Geometry: see drawing. Coordinates: mm, zero at the bounding-box minimum. A direction names the side the tool comes from. Coordinates: 2 decimals unless noted, no trailing zeros. Loops run counter-clockwise (first coordinate to the right, second up) from the corner with the lowest first, then second, coordinate; pieces in that order, holes last.
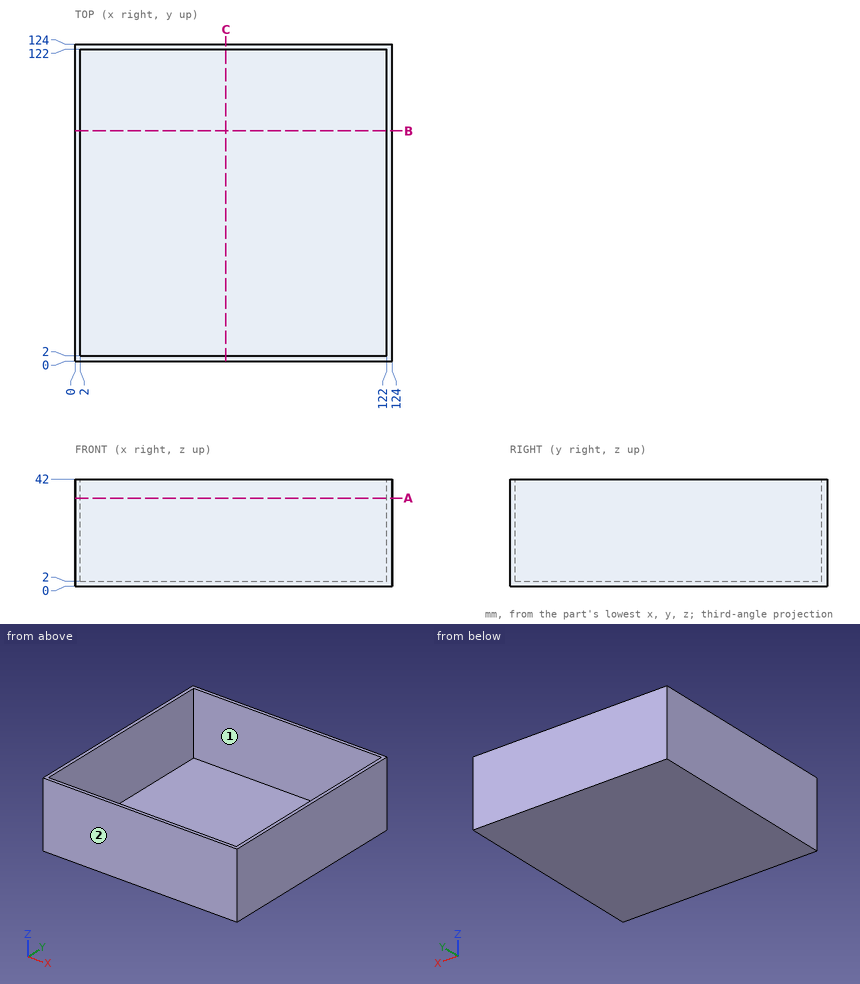
Item 1: Reachability of the marked faces 1 and 2 from +Z, -Z, +X, -X, +Y, -Y: full face, straight path, thin tool, end or side. Return the list, or none.
Result:
face 1: +Z
face 2: +Z, -Z, +X, -X, -Y
Item 2: Section query A-A (z = 34.5). Output: boundary loops of the cut face in (x, y), then the cut area to 3 significant figures.
Result:
outline: (0, 0) - (124, 0) - (124, 124) - (0, 124) - close; hole (2, 2) - (122, 2) - (122, 122) - (2, 122) - close
area: 976 mm2
Item 3: Section query B-B (y = 90). Output: boundary loops of the cut face in (x, z), then the cut area to 3 significant figures.
Result:
outline: (0, 0) - (124, 0) - (124, 42) - (122, 42) - (122, 2) - (2, 2) - (2, 42) - (0, 42) - close
area: 408 mm2
Item 4: Contact query for flat-ended pins moving along their axis: P1, Ø12, axis at y = 45.5, z = 17.5, coming from the -X side; P2, Ø4, axis at x = 104, y = 18.5, coming from the +Z side. Output: stop coordinate, or through.
Result:
P1: stops at x = 0
P2: stops at z = 2
Item 5: Line query: L1, parallel to X at y = 78, z = 23.5; L2, parallel to Z at x = 111, y = 9. Output: solid intervals per line, ascending.
Result:
L1: x = 0 to 2, 122 to 124
L2: z = 0 to 2
